Geometry: see drawing. Coordinates: mm, zero at the bounding-box minimum. A direction names the side the tool comes from. Coordinates: 2 decimals unless noted, no trailing zeros. Order: outer loops, then holes, each group sorted by start corner. A loop starts at its lowest first (then second) coordinate and runs counter-clockwise, first axis right, second up.
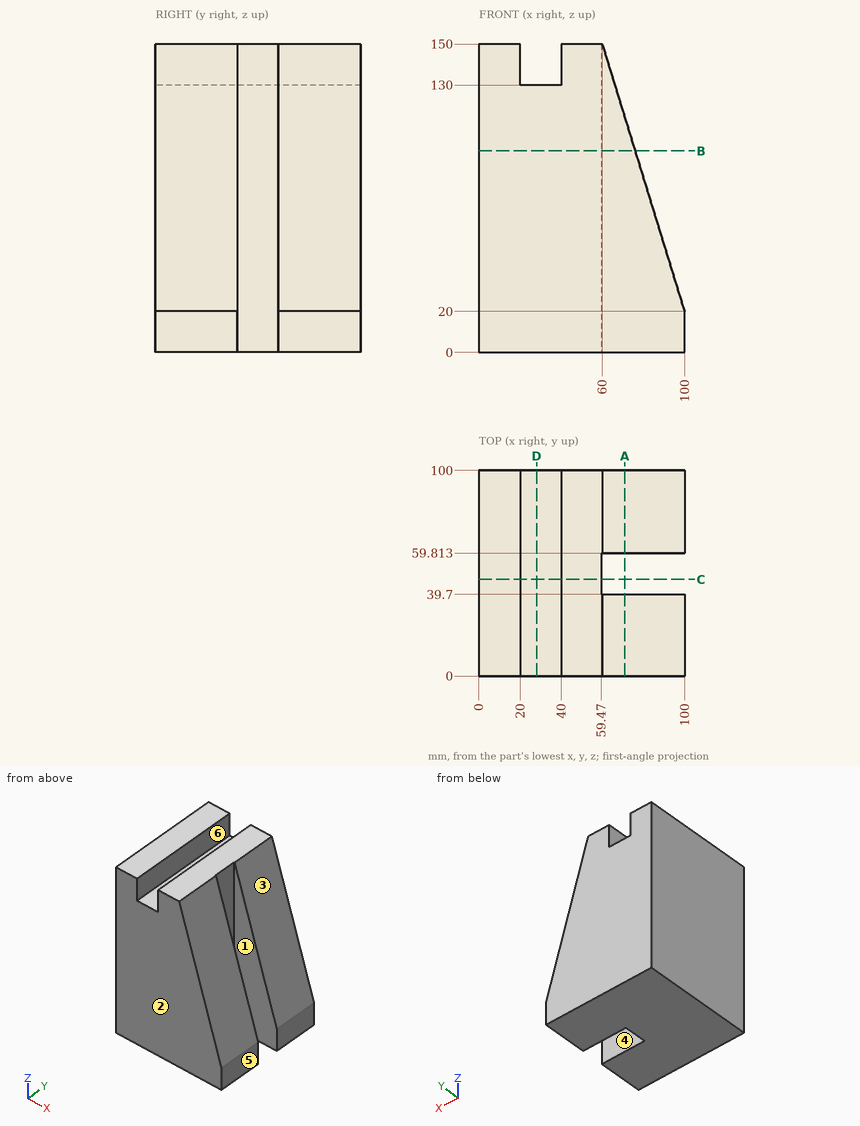
Q1. Pull-direction query (Y, two-part tool) for the marked faces 1, 2 and 3; classes: pulls with the +Y half, pulls with the -Y half, needs draft (parallel to the pull), parting line crosses it, or undercut.
Solutions:
face 1: undercut
face 2: pulls with the -Y half
face 3: needs draft
Q2. Material intervals for line 1 along Y through (x, z) = (69, 36.5); line 2 along Z through (x, y) = (32.5, 17.5); line 3 along X through (y, z) = (26, 140), sorted ascending.
Solutions:
line 1: y = 0 to 39.7, 59.81 to 100
line 2: z = 0 to 130
line 3: x = 0 to 20, 40 to 63.08
Q3. Section query C-C on y = 47. Output: boundary loops of the cut face in (x, z).
Solutions:
outline: (0, 0) - (59.47, 0) - (59.47, 150) - (40, 150) - (40, 130) - (20, 130) - (20, 150) - (0, 150) - close
Q4. Section query B-B on z = 98. Output: boundary loops of the cut face in (x, y), plus the area to 3 significant figures.
Solutions:
outline: (0, 0) - (76, 0) - (76, 39.7) - (59.47, 39.7) - (59.47, 59.81) - (76, 59.81) - (76, 100) - (0, 100) - close
area: 7,270 mm2
Q5. Section query D-D on x = 28. Output: boundary loops of the cut face in (y, z), plus the area to 3 significant figures.
Solutions:
outline: (0, 0) - (100, 0) - (100, 130) - (0, 130) - close
area: 13,000 mm2
Q6. Set-up query: the marked faces 4, 5 and 6. Return all of +Z, -Z, +X, -X, +Y, -Y with unobstructed straight access to the full face (end or side cutting, diameter ignored); none if empty.
Solutions:
face 4: +Z, -Z, +X
face 5: +Z, -Z, +X, +Y, -Y
face 6: +Z, +Y, -Y
Q7. Section query A-A on x = 71. Output: boundary loops of the cut face in (y, z).
Solutions:
outline: (0, 0) - (39.7, 0) - (39.7, 114.25) - (0, 114.25) - close; (59.81, 0) - (100, 0) - (100, 114.25) - (59.81, 114.25) - close
Q8. Pin query (flat end, axial travel): P1, Ø6, axis at y = 52.5, z = 62.5, coming from the +X side; P2, Ø16, axis at y = 75, z = 135.5, coming from the +X side; P3, Ø6, axis at x = 26, y = 50, coming from the +Z side. Return the tip coordinate at first contact, or that it passes through.
Solutions:
P1: stops at x = 59.47
P2: stops at x = 66.92
P3: stops at z = 130
